from build123d import *

# Parameters (mm, degrees)
SKETCH_2_W          = 80
SKETCH_2_H          = 140
EXTRUDE_1_DEPTH     = 4
SKETCH_3_R          = 1.8
SKETCH_3_R_2        = 2.35
SKETCH_3_R_3        = 2.5
CUT_EXTRUDE_3_DEPTH = 4
CUT_EXTRUDE_4_REACH = 108.377
SKETCH_4_W          = 20
SKETCH_4_H          = 50


with BuildPart() as part:
    # 草图2 → 凸台-拉伸1 (new body)
    with BuildSketch(Plane(origin=(0, 0, 0), x_dir=(1, 0, 0), z_dir=(0, 1, 0))):
        with Locations((-40, 0)):
            Rectangle(SKETCH_2_W, SKETCH_2_H)
    extrude(amount=EXTRUDE_1_DEPTH)

    # 草图3 → 切除-拉伸3 (cut)
    with BuildSketch(Plane(origin=(0, 4, 0), x_dir=(1, 0, 0), z_dir=(0, 1, 0))):
        with Locations(Location((-72, 63.5, 0), (0, 0, 270))):
            Circle(SKETCH_3_R)
        with Locations(Location((-41, 63.5, 0), (0, 0, 270))):
            Circle(SKETCH_3_R)
        with Locations(Location((-41, 36.5, 0), (0, 0, 270))):
            Circle(SKETCH_3_R)
        with Locations(Location((-72, 36.5, 0), (0, 0, 270))):
            Circle(SKETCH_3_R)
        with Locations(Location((-41, -63.5, 0), (0, 0, 270))):
            Circle(SKETCH_3_R)
        with Locations(Location((-41, -36.5, 0), (0, 0, 270))):
            Circle(SKETCH_3_R)
        with Locations(Location((-72, -36.5, 0), (0, 0, 270))):
            Circle(SKETCH_3_R)
        with Locations(Location((-72, -63.5, 0), (0, 0, 270))):
            Circle(SKETCH_3_R)
        with Locations(Location((-73.9, 50, 0), (0, 0, 270))):
            Circle(SKETCH_3_R_2)
        with Locations(Location((-73.9, -50, 0), (0, 0, 270))):
            Circle(SKETCH_3_R_2)
        with Locations(Location((-39.1, -50, 0), (0, 0, 270))):
            Circle(SKETCH_3_R_2)
        with Locations(Location((-39.1, 50, 0), (0, 0, 270))):
            Circle(SKETCH_3_R_2)
        with Locations(Location((-10, 60, 0), (0, 0, 270))):
            Circle(SKETCH_3_R_3)
        with Locations(Location((-10, 0, 0), (0, 0, 270))):
            Circle(SKETCH_3_R_3)
        with Locations(Location((-10, -60, 0), (0, 0, 270))):
            Circle(SKETCH_3_R_3)
    extrude(amount=-CUT_EXTRUDE_3_DEPTH, mode=Mode.SUBTRACT)

    # 草图4 → 切除-拉伸4 (cut, up to next)
    with BuildSketch(Plane.XZ, mode=Mode.PRIVATE) as cut_extrude_4_sk1:
        with Locations((-28.074591113, 0.884472787)):
            Rectangle(SKETCH_4_W, SKETCH_4_H)
    cut_extrude_4_tool1 = extrude(cut_extrude_4_sk1.sketch, amount=-CUT_EXTRUDE_4_REACH, mode=Mode.PRIVATE) & part.part
    add(cut_extrude_4_tool1.solids().sort_by_distance((-28.074591, 0, 0.884473))[0], mode=Mode.SUBTRACT)


solid = part.part
Read the model definition and answer for the solid it produces. Units are mm, in the model's axes. A direction names the side the tool comes from. Round coordinates to 2 decimals unless told otherwise and drop trailing zeros. Loops run counter-clockwise (first coordinate to the right, second up) from the corner with the lowest first, then second, coordinate; pieces in that order, holes last.
Q1. Consider probe 1 along X at (y, z) = (2.2, -36.5); probe 2 along X at (y, z) = (3.1, 50); probe 3 along X at (y, z) = (1.4, 23). Determine where each line is inside the solid, lowest interval first.
Q2. Section A-A on z = 60 is taken. Write down the section's boundary in (x, y), and give its area (3 significant figures).
Q3. Section D-D on z = -36.5 is taken. Write down the section's boundary in (x, y), and give its area (3 significant figures).
Q4. Determine the mould class of faces 1 (the face through (-38.075, 2, 1)), 2 (the face through (0, 2, 1)), 3 (the face through (-39.783, 2.028, -64.827)) for opening direction Z: released by +Z, released by -Z, zero draft, split by the parting line, or undercut.
Q5. Which of the six approach directions +Z, -Z, +X, -X, +Y, -Y give full straight-line access (tool end or side, diameter ignored) to faces 4 (the face through (-41, 4, -1)), 5 (the face through (-28, 2, 25.884))?
Q6. Section C-C on y = 3.1 is taken. Give the number of separate pieces and of enclosed holes in the cut face, and give its area (3 significant figures).
Q7. Section B-B on x = -19.5 is taken. Write down the section's boundary in (y, z).
Output:
1. probe 1: x = -80 to -73.8, -70.2 to -42.8, -39.2 to 0
1. probe 2: x = -80 to -76.25, -71.55 to -41.45, -36.75 to 0
1. probe 3: x = -80 to -38.07, -18.07 to 0
2. outline: (-80, 0) - (-12.5, 0) - (-12.5, 4) - (-80, 4) - close; (-7.5, 0) - (0, 0) - (0, 4) - (-7.5, 4) - close
2. area: 300 mm2
3. outline: (-80, 0) - (-73.8, 0) - (-73.8, 4) - (-80, 4) - close; (-70.2, 0) - (-42.8, 0) - (-42.8, 4) - (-70.2, 4) - close; (-39.2, 0) - (0, 0) - (0, 4) - (-39.2, 4) - close
3. area: 291 mm2
4. face 1: undercut
4. face 2: zero draft
4. face 3: undercut
5. face 4: +Z, -Z, +X, -X, +Y
5. face 5: +Y, -Y
6. separate pieces: 1
6. enclosed holes: 16
6. area: 9,990 mm2
7. outline: (0, -70) - (4, -70) - (4, -24.12) - (0, -24.12) - close; (0, 25.88) - (4, 25.88) - (4, 70) - (0, 70) - close
